from build123d import *

# Parameters (mm, degrees)
F1_DEPTH = 5
F2_DEPTH = 20
F3_R     = 13
F4_DEPTH = 25
F5_R     = 5.5
F6_DEPTH = 25


with BuildPart() as f1:
    # F0 (on Front) → F1 (new body)
    with BuildSketch(Plane.XZ):
        Polygon((23.6713610368, -41), (47.3427220735, 0), (23.6713610368, 41), (-23.6713610368, 41), (-47.3427220735, 0), (-23.6713610368, -41), align=None)
        Polygon((20.7846096908, 36), (41.5692193817, 0), (20.7846096908, -36), (-20.7846096908, -36), (-41.5692193817, 0), (-20.7846096908, 36), align=None, mode=Mode.SUBTRACT)
        Polygon((20.7846096908, -36), (41.5692193817, 0), (20.7846096908, 36), (-20.7846096908, 36), (-41.5692193817, 0), (-20.7846096908, -36), align=None)
    extrude(amount=-F1_DEPTH)

    # F0 (on Front) → F2 (join)
    with BuildSketch(Plane.XZ):
        Polygon((23.6713610368, -41), (47.3427220735, 0), (23.6713610368, 41), (-23.6713610368, 41), (-47.3427220735, 0), (-23.6713610368, -41), align=None)
        Polygon((20.7846096908, 36), (41.5692193817, 0), (20.7846096908, -36), (-20.7846096908, -36), (-41.5692193817, 0), (-20.7846096908, 36), align=None, mode=Mode.SUBTRACT)
    extrude(amount=F2_DEPTH)

    # F3 (on face) → F4 (cut)
    with BuildSketch(Plane.XZ):
        Circle(F3_R)
    extrude(amount=-F4_DEPTH, mode=Mode.SUBTRACT)

    # F5 (on face) → F6 (cut)
    with BuildSketch(Plane.XZ):
        with Locations((29.2692193817, 0)):
            Circle(F5_R)
        with Locations((-29.2692193817, 0)):
            Circle(F5_R)
    extrude(amount=-F6_DEPTH, mode=Mode.SUBTRACT)


solid = f1.part
Check sheet for the modelled part. Datum: model origin and axes. Units: mm. A direction names the side the tool comes from. Coordinates: 2 decimals unless noted, no trailing zeros. Write each loop counter-clockwise with the first axis right and the second up, starting at its lowest first coordinate (ties: lowest second). Pieces come first, ordered by that corner, then holes.
Item 1: Mould release check, pull along Z, two halves, no side actions. Record for faces 3 (the face through (18, 0, 1)), 4 (the face through (-35.673, -7.325, -20.213)), 5 (the face through (35.673, -7.325, 20.213)): released by +Z, released by -Z, zero draft, split by the parting line, or undercut.
Numbers:
face 3: undercut
face 4: released by -Z
face 5: released by +Z
Item 2: Access from +Z, -Z, +X, -X, +Y, -Y to the whole of each face (thin tool, end or side, straight path). Record for faces 1 (the face through (0, -7, -41)), 2 (the face through (31.031, -9.86, 18.252)).
Numbers:
face 1: -Z, +X, -X, +Y, -Y
face 2: -Y
Item 3: Cross-section at A-A on y = -12.75. Record the boundary of the cut face in (x, z).
Numbers:
outline: (-47.34, 0) - (-23.67, -41) - (23.67, -41) - (47.34, 0) - (23.67, 41) - (-23.67, 41) - close; hole (-41.57, 0) - (-20.78, -36) - (20.78, -36) - (41.57, 0) - (20.78, 36) - (-20.78, 36) - close
Item 4: Cross-section at B-B on x = 0. Record the boundary of the cut face in (y, z), then the cut area to 3 significant figures.
Numbers:
outline: (-20, -41) - (5, -41) - (5, -13) - (0, -13) - (0, -36) - (-20, -36) - close; (-20, 36) - (0, 36) - (0, 13) - (5, 13) - (5, 41) - (-20, 41) - close
area: 480 mm2
Item 5: Scan lines: probe 1 along Z at (x, y) = (13, -14.75); probe 2 along Z at (x, y) = (0, 3.8); probe 3 along Y at (x, z) = (19, 19). Record each from-to range of solid material in increasing order.
Numbers:
probe 1: z = -41 to -36, 36 to 41
probe 2: z = -41 to -13, 13 to 41
probe 3: y = 0 to 5
Item 6: Cross-section at C-C on x = 16.5. Record the boundary of the cut face in (y, z), then the cut area to 3 significant figures.
Numbers:
outline: (-20, -41) - (5, -41) - (5, 41) - (-20, 41) - (-20, 36) - (0, 36) - (0, -36) - (-20, -36) - close
area: 610 mm2
Item 7: Cross-section at D-D on z = 20. Record the boundary of the cut face in (x, y), then the cut area to 3 significant figures.
Numbers:
outline: (-35.8, -20) - (-30.02, -20) - (-30.02, 0) - (30.02, 0) - (30.02, -20) - (35.8, -20) - (35.8, 5) - (-35.8, 5) - close
area: 589 mm2
Item 8: Depth check by flat-ended pin: pin 1 Ø8 at (x, z) = (1, -10.5) entering from -Y; pin 2 Ø5 at (y, z) = (-2, 32.5) entering from +X; pin 3 Ø8 at (y, z) = (-10, 12.5) entering from +X. Enter the tip coordinate at first touch or a pass-through.
Numbers:
pin 1: stops at y = 0
pin 2: stops at x = 30.02
pin 3: stops at x = 42.44
